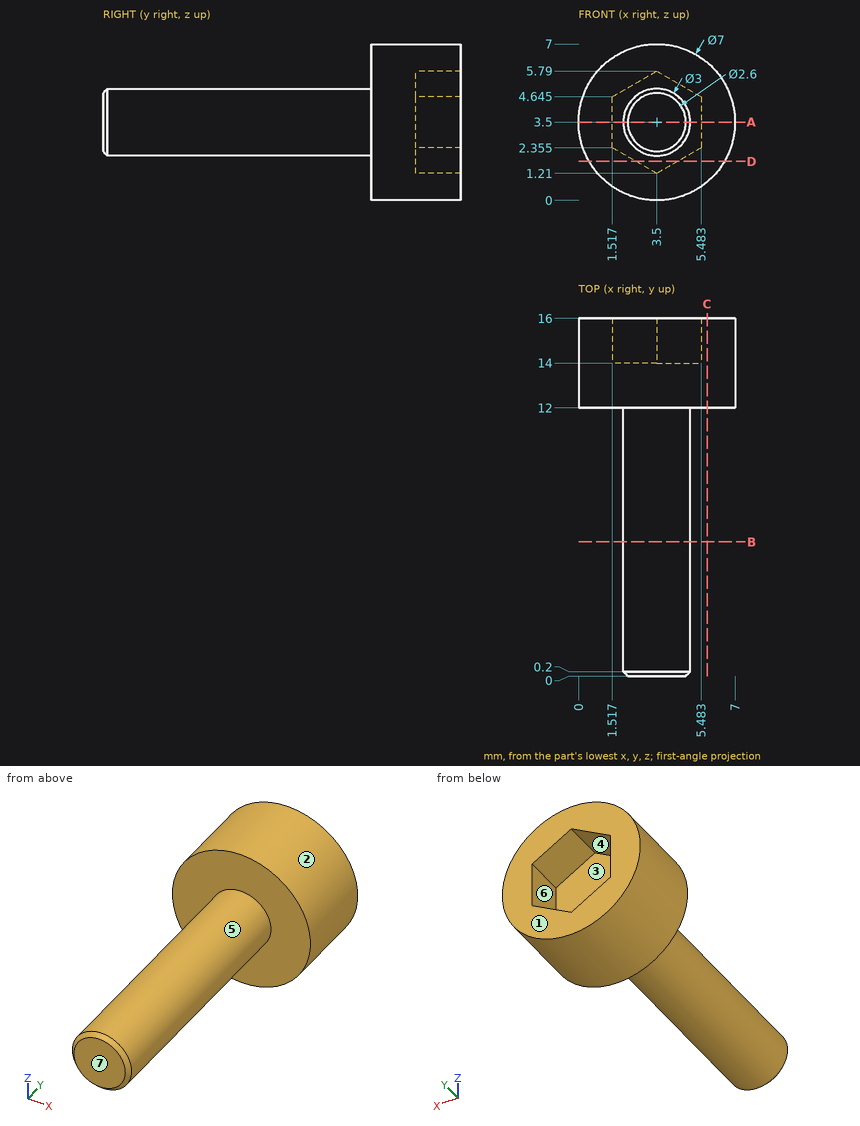
The figure shows three views and two pictorial views of one solid part (mm, origin at its lowest corner). Answer the questions. A direction names the side the tool comes from. Coordinates: 2 decimals unless noted, no trailing zeros. Write each loop counter-clockwise with the first axis right and the second up, starting at its lowest first coordinate (ties: lowest second). Pieces come first, ordered by that corner, then holes.
1. Flat-ended cylindrical pins translate along their axes: pin 1 (4 mm diameter, centred on y = 7, z = 4.5, fed in from +X); pin 2 (2 mm diameter, centred on x = 1, z = 6, fed in from -Y); pin 3 (0.6 mm diameter, centred on y = 15, z = 4, fed in from +X). Find the tip coordinate at first contact, or state that the pin passes through.
Results list:
pin 1: stops at x = 5
pin 2: stops at y = 12
pin 3: stops at x = 6.99
2. For the marked faces 5, 6 and 7, determine the directions among +Z, -Z, +X, -X, +Y, -Y from which every point of the face is accessible in a straight line to the end or side of a thin tool.
Results list:
face 5: -Y
face 6: +Y
face 7: +Z, -Z, +X, -X, -Y
3. The part is cut by section D-D, the plane z = 1.75. Write down the section's boundary in (x, y) (1 decimal), and give its area (3 significant figures).
Results list:
outline: (0.5, 12) - (6.5, 12) - (6.5, 16) - (4.4, 16) - (4.4, 14) - (2.6, 14) - (2.6, 16) - (0.5, 16) - close
area: 20.5 mm2
4. The part is cut by section A-A, the plane z = 3.5. Write down the section's boundary in (x, y).
Results list:
outline: (0, 12) - (2, 12) - (2, 0.2) - (2.2, 0) - (4.8, 0) - (5, 0.2) - (5, 12) - (7, 12) - (7, 16) - (5.48, 16) - (5.48, 14) - (1.52, 14) - (1.52, 16) - (0, 16) - close
5. The part is cut by section C-C, the plane x = 5.75. Write down the section's boundary in (y, z).
Results list:
outline: (12, 0.82) - (16, 0.82) - (16, 6.18) - (12, 6.18) - close
6. Consider line 1 along Y through (x, z) = (0.75, 2.75); line 2 along Y through (x, z) = (5, 4.5); line 3 along Z through (x, y) = (2.25, 14.75). Determine where each line is inside the solid, lowest interval first.
Results list:
line 1: y = 12 to 16
line 2: y = 12 to 14
line 3: z = 0.23 to 1.93, 5.07 to 6.77
7. For a pull along Z with two mould halves and no side action, classify the marked faces 1, 2, 3 and 4 as +Z half, -Z half, draft (parallel to the pull), parting line (faces both ways), or undercut.
Results list:
face 1: draft
face 2: parting line
face 3: undercut
face 4: undercut
8. The part is cut by section B-B, the plane y = 6. Write down the section's boundary in (x, z).
Results list:
outline: circle Ø3 at (3.5, 3.5)
